from build123d import *

# Parameters (mm, degrees)
SKETCH1_W                   = 100
SKETCH1_H                   = 100
SKETCH1_W_2                 = 45.4
SKETCH1_H_2                 = 45.4
BOSS_EXTRUDE1_DEPTH         = 24
FILLET1_R                   = 3
SKETCH2_W                   = 100
SKETCH2_H                   = 100
BOSS_EXTRUDE2_DEPTH         = 6
SKETCH3_W                   = 100
SKETCH3_H                   = 100
SKETCH3_W_2                 = 96.8
SKETCH3_H_2                 = 96.8
CUT_EXTRUDE1_DEPTH          = 7
SKETCH4_R                   = 1.1305
CUT_EXTRUDE2_DEPTH          = 4.7
SKETCH5_W                   = 100
SKETCH5_H                   = 100
SKETCH5_W_2                 = 96.6
SKETCH5_H_2                 = 96.6
BOSS_EXTRUDE3_DEPTH         = 13
FILLET2_R                   = 3
SKETCH6_R                   = 5.5
CUT_EXTRUDE3_DEPTH          = 80.806014811
F_32_0_116_DIAMETER_HOLE1_D = 2.9464
F_32_0_116_DIAMETER_HOLE2_D = 2.9464
F_4_40_TAPPED_HOLE1_D       = 2.2606
F_4_40_TAPPED_HOLE1_DEPTH   = 8.86
F_4_40_TAPPED_HOLE1_TIP     = 0.679152758
F_4_40_TAPPED_HOLE2_D       = 2.2606
F_4_40_TAPPED_HOLE2_DEPTH   = 8.87
F_4_40_TAPPED_HOLE2_TIP     = 0.679152758
F_4_40_TAPPED_HOLE3_D       = 2.2606
F_4_40_TAPPED_HOLE3_DEPTH   = 8.87
F_4_40_TAPPED_HOLE3_TIP     = 0.679152758
F_4_40_TAPPED_HOLE4_D       = 2.2606
F_4_40_TAPPED_HOLE4_DEPTH   = 8.87
F_4_40_TAPPED_HOLE4_TIP     = 0.679152758


with BuildPart() as part:
    # Sketch1 → Boss-Extrude1 (new body)
    with BuildSketch(Plane(origin=(0, 0, 0), x_dir=(1, 0, 0), z_dir=(0, 1, 0))):
        Rectangle(SKETCH1_W, SKETCH1_H)
        with Locations((-23.3, -23.3)):
            Rectangle(SKETCH1_W_2, SKETCH1_H_2, mode=Mode.SUBTRACT)
        with Locations((-23.3, 23.3)):
            Rectangle(SKETCH1_W_2, SKETCH1_H_2, mode=Mode.SUBTRACT)
        with Locations((23.3, -23.3)):
            Rectangle(SKETCH1_W_2, SKETCH1_H_2, mode=Mode.SUBTRACT)
        with Locations((23.3, 23.3)):
            Rectangle(SKETCH1_W_2, SKETCH1_H_2, mode=Mode.SUBTRACT)
    extrude(amount=BOSS_EXTRUDE1_DEPTH)

    # Fillet1
    fillet1_edges = [part.edges().sort_by_distance(p)[0] for p in [
        (-46, 12, 46),
        (-0.6, 12, 46),
        (-0.6, 12, 0.6),
        (-46, 12, 0.6),
        (-46, 12, -46),
        (-46, 12, -0.6),
        (-0.6, 12, -0.6),
        (-0.6, 12, -46),
        (46, 12, -0.6),
        (46, 12, -46),
        (0.6, 12, -46),
        (0.6, 12, -0.6),
        (0.6, 12, 46),
        (46, 12, 46),
        (46, 12, 0.6),
        (0.6, 12, 0.6),
    ]]
    fillet(fillet1_edges, radius=FILLET1_R)

    # Sketch2 → Boss-Extrude2 (add)
    with BuildSketch(Plane.XZ):
        Rectangle(SKETCH2_W, SKETCH2_H)
    extrude(amount=BOSS_EXTRUDE2_DEPTH)

    # Sketch3 → Cut-Extrude1 (cut)
    with BuildSketch(Plane.XZ.offset(6)):
        Rectangle(SKETCH3_W, SKETCH3_H)
        Rectangle(SKETCH3_W_2, SKETCH3_H_2, mode=Mode.SUBTRACT)
    extrude(amount=-CUT_EXTRUDE1_DEPTH, mode=Mode.SUBTRACT)

    # Sketch4 → Cut-Extrude2 (cut)
    with BuildSketch(Plane.XZ.offset(6)):
        with Locations(Location((42.865, -40.005, 0), (0, 0, 270))):
            Circle(SKETCH4_R)
        with Locations(Location((-42.865, -37.465, 0), (0, 0, 270))):
            Circle(SKETCH4_R)
        with Locations(Location((42.865, 40.005, 0), (0, 0, 270))):
            Circle(SKETCH4_R)
        with Locations(Location((-42.865, 36.195, 0), (0, 0, 270))):
            Circle(SKETCH4_R)
    extrude(amount=-CUT_EXTRUDE2_DEPTH, mode=Mode.SUBTRACT)

    # Sketch5 → Boss-Extrude3 (add)
    with BuildSketch(Plane(origin=(0, 24, 0), x_dir=(1, 0, 0), z_dir=(0, 1, 0))):
        Rectangle(SKETCH5_W, SKETCH5_H)
        Rectangle(SKETCH5_W_2, SKETCH5_H_2, mode=Mode.SUBTRACT)
    extrude(amount=BOSS_EXTRUDE3_DEPTH)

    # Fillet2
    fillet2_edges = [part.edges().sort_by_distance(p)[0] for p in [
        (-48.4, -2.5, -48.4),
        (-48.4, -2.5, 48.4),
        (48.4, -2.5, 48.4),
        (48.4, -2.5, -48.4),
        (48.3, 30.5, 48.3),
        (48.3, 30.5, -48.3),
        (-48.3, 30.5, -48.3),
        (-48.3, 30.5, 48.3),
    ]]
    fillet(fillet2_edges, radius=FILLET2_R)

    # Sketch6 → Cut-Extrude3 (cut, through all)
    with BuildSketch(Plane(origin=(0, 0, 0), x_dir=(1, 0, 0), z_dir=(0, 1, 0))):
        with Locations(Location((-23.3, 23.3, 0), (0, 0, 270))):
            Circle(SKETCH6_R)
        with Locations(Location((23.3, 23.3, 0), (0, 0, 270))):
            Circle(SKETCH6_R)
        with Locations(Location((23.3, -23.3, 0), (0, 0, 270))):
            Circle(SKETCH6_R)
        with Locations(Location((-23.3, -23.3, 0), (0, 0, 270))):
            Circle(SKETCH6_R)
    extrude(amount=-CUT_EXTRUDE3_DEPTH, mode=Mode.SUBTRACT)

    # #32 (0.116) Diameter Hole1 (through all)
    with Locations(Plane.XY.offset(50)):
        with Locations((0, 32), (-37.55, 32), (37.55, 32)):
            Hole(F_32_0_116_DIAMETER_HOLE1_D / 2)

    # #32 (0.116) Diameter Hole2 (through all)
    with Locations(Plane(origin=(50, 0, 0), x_dir=(0, 0, -1), z_dir=(1, 0, 0))):
        with Locations((0, 32), (-37.55, 32), (37.55, 32)):
            Hole(F_32_0_116_DIAMETER_HOLE2_D / 2)

    # #4-40 Tapped Hole1
    with Locations(Plane(origin=(0, 0, -48.4), x_dir=(-1, 0, 0), z_dir=(0, 0, -1))):
        with Locations((-30, -3), (30, -3)):
            Hole(F_4_40_TAPPED_HOLE1_D / 2, depth=F_4_40_TAPPED_HOLE1_DEPTH)
            with Locations((0, 0, -(F_4_40_TAPPED_HOLE1_DEPTH + F_4_40_TAPPED_HOLE1_TIP / 2))):  # 118° drill point
                Cone(0, F_4_40_TAPPED_HOLE1_D / 2, F_4_40_TAPPED_HOLE1_TIP, mode=Mode.SUBTRACT)

    # #4-40 Tapped Hole2
    with Locations(Plane(origin=(48.4, 0, 0), x_dir=(0, 0, -1), z_dir=(1, 0, 0))):
        with Locations((-30, -3), (30, -3)):
            Hole(F_4_40_TAPPED_HOLE2_D / 2, depth=F_4_40_TAPPED_HOLE2_DEPTH)
            with Locations((0, 0, -(F_4_40_TAPPED_HOLE2_DEPTH + F_4_40_TAPPED_HOLE2_TIP / 2))):  # 118° drill point
                Cone(0, F_4_40_TAPPED_HOLE2_D / 2, F_4_40_TAPPED_HOLE2_TIP, mode=Mode.SUBTRACT)

    # #4-40 Tapped Hole3
    with Locations(Plane.XY.offset(48.4)):
        with Locations((-30, -3), (30, -3)):
            Hole(F_4_40_TAPPED_HOLE3_D / 2, depth=F_4_40_TAPPED_HOLE3_DEPTH)
            with Locations((0, 0, -(F_4_40_TAPPED_HOLE3_DEPTH + F_4_40_TAPPED_HOLE3_TIP / 2))):  # 118° drill point
                Cone(0, F_4_40_TAPPED_HOLE3_D / 2, F_4_40_TAPPED_HOLE3_TIP, mode=Mode.SUBTRACT)

    # #4-40 Tapped Hole4
    with Locations(Plane.ZY.offset(48.4)):
        with Locations((-30, -3), (30, -3)):
            Hole(F_4_40_TAPPED_HOLE4_D / 2, depth=F_4_40_TAPPED_HOLE4_DEPTH)
            with Locations((0, 0, -(F_4_40_TAPPED_HOLE4_DEPTH + F_4_40_TAPPED_HOLE4_TIP / 2))):  # 118° drill point
                Cone(0, F_4_40_TAPPED_HOLE4_D / 2, F_4_40_TAPPED_HOLE4_TIP, mode=Mode.SUBTRACT)


solid = part.part
Design review of the part built by this model. Coordinates are the model's own, in mm. A direction names the side the tool comes from. Give positions to 0.01 mm unless a question says otherwise; leave off trailing zeros. Write each loop counter-clockwise with the first axis right and the second up, starting at its lowest first coordinate (ties: lowest second). Pieces come first, ordered by that corner, then holes. Notation, with made-up numbers: M 26,5 L 37,5 A24 ccw 37,39 Z; hole C -7,19 d10. An arc over 180 degrees is marked long. Answer as a JSON object with one key per item and string values. Group by question number.
1) We need section A-A (x = -37.55). Give the boundary of the cut face in (y, z).
2) Tool access review of faces 4 (the face through (-47.54, -2.45, -47.5)), 5 (the face through (-31.13, -2.95, -43.91)), 6 (the face through (0, 24, 0)): name each direction out of +Z, -Z, +X, -X, +Y, -Y from which nothing blocks a thin tool from reaching the whole face with its end or side.
3) We need section C-C (z = -12.5). Give the boundary of the cut face in (x, y).
4) Mouldability with a two-part tool opening along Z and no side actions: class faces 1 (the face through (29.81, -2.94, -38.98)), 2 (the face through (49.138, 31.436, 38.911)), 3 (the face through (-38.911, 31.436, 49.138)) as released by +Z, released by -Z, zero draft, split by the parting line, or undercut.
5) We need section B-B (z = 27). Give the boundary of the cut face in (x, y).
6) For line 1 along Z through (x, y) = (-29, 3); line 2 along X through (y, z) = (-1.7, 23.3), list the stretches that pass through material, from the lowest coordinate up.
7) Clearance check with flat-ended pins moving along their axes: pin 1 Ø2 at (x, y) = (30, -3) entering from +Z; pin 2 Ø1.4 at (x, z) = (-42.865, -37.465) entering from -Y; pin 3 Ø22.5 at (x, z) = (-21, 12.5) entering from +Y; pin 4 Ø4.5 at (x, y) = (37.55, 32) entering from +Z. State where each tip first meets the part, or that it passes through.
8) We need section D-D (y = 32). Count the separate pieces of the cut face and the enclosed holes in it, and give its area (3 significant figures).
Answer key:
{
 "1": {"outline": "M -6,-48.4 L 1,-48.4 L 1,-50 L 30.53,-50 L 30.53,-48.3 L 24,-48.3 L 24,-46 L 0,-46 L 0,-0.6 L 24,-0.6 L 24,0.6 L 0,0.6 L 0,46 L 24,46 L 24,48.3 L 30.53,48.3 L 30.53,50 L 1,50 L 1,48.4 L -6,48.4 Z; M 33.47,-50 L 37,-50 L 37,-48.3 L 33.47,-48.3 Z; M 33.47,48.3 L 37,48.3 L 37,50 L 33.47,50 Z"},
 "2": {"face 4": "-Z, -X, -Y", "face 5": "-Z", "face 6": "+Y"},
 "3": {"outline": "M -50,1 L -48.4,1 L -48.4,-6 L 48.4,-6 L 48.4,1 L 50,1 L 50,37 L 48.3,37 L 48.3,24 L 46,24 L 46,0 L 0.6,0 L 0.6,24 L -0.6,24 L -0.6,0 L -46,0 L -46,24 L -48.3,24 L -48.3,37 L -50,37 Z"},
 "4": {"face 1": "released by -Z", "face 2": "undercut", "face 3": "zero draft"},
 "5": {"outline": "M -50,1 L -48.4,1 L -48.4,-6 L -27.37,-6 L -27.37,0 L -46,0 L -46,24 L -48.3,24 L -48.3,37 L -50,37 Z; M -19.23,-6 L 19.23,-6 L 19.23,0 L 0.6,0 L 0.6,24 L -0.6,24 L -0.6,0 L -19.23,0 Z; M 27.37,-6 L 48.4,-6 L 48.4,1 L 50,1 L 50,37 L 48.3,37 L 48.3,24 L 46,24 L 46,0 L 27.37,0 Z"},
 "6": {"line 1": "z = -50 to -46, -0.6 to 0.6, 46 to 50", "line 2": "x = -48.4 to -28.8, -17.8 to 17.8, 28.8 to 48.4"},
 "7": {"pin 1": "stops at z = 39.45", "pin 2": "stops at y = -1.3", "pin 3": "stops at y = 0", "pin 4": "stops at z = 50"},
 "8": {"separate pieces": "12", "enclosed holes": "0", "area": "616 mm²"}
}
